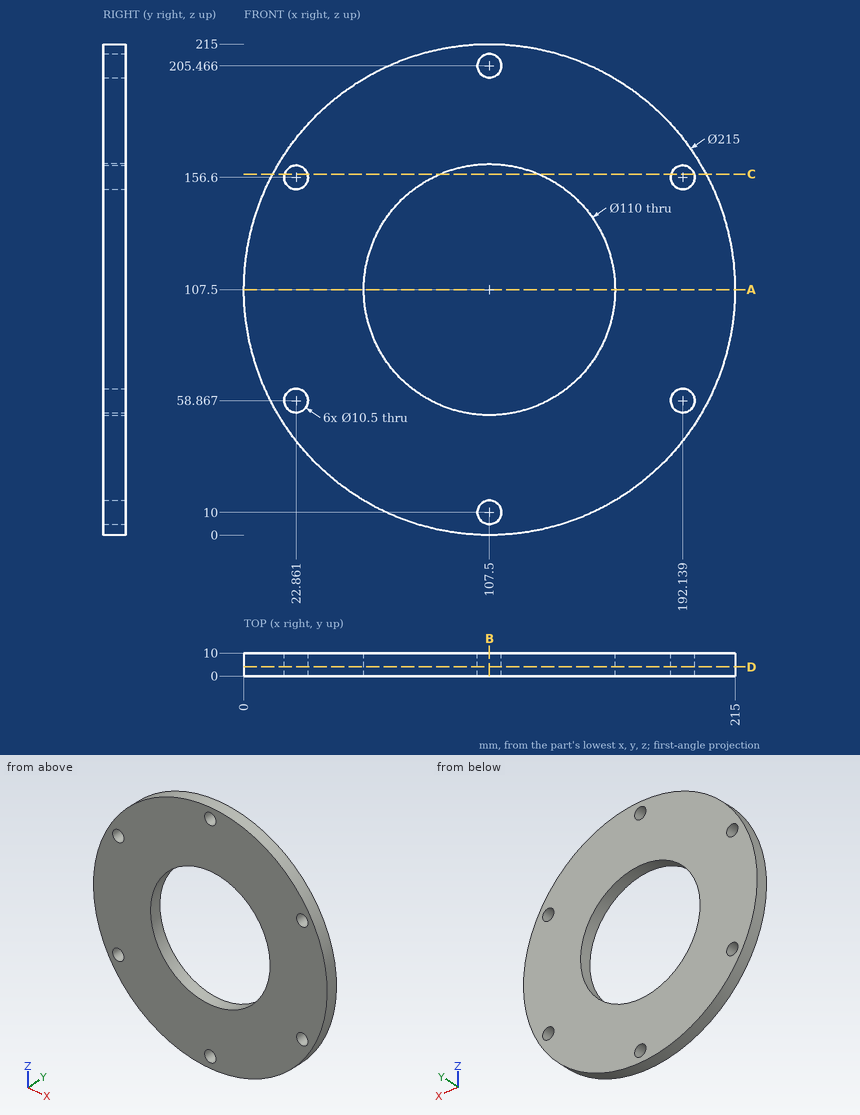
Here's the drawing with two shaded views (mm, measured from the low corner). I have some questions. Give positions to 0.01 mm unless a question says otherwise; leave off trailing zeros. Order: outer loops, then holes, each group sorted by start corner. A loop starts at its lowest first (then second) coordinate and runs counter-clockwise, first axis right, second up. Notation, with made-up numbers: (-2.75, 20) - (25.25, 20) arc R16 cw to (25.25, 43) - close; hole circle Ø5 at (29.5, 56). An arc over 180 degrees is marked (long way). Use a Markdown table: item, result. Add a question column.
Q1. If we section it at D-D on y = 4: Count the separate pieces of the cut face and the enclosed holes in it, plus the area to 3 significant figures.
Q2. I'm going to push flat-ended pins straight in: pin 1 (6 mm diameter, centred on x = 101.5, y = 7.5, fed in from -Z); pin 2 (1 mm diameter, centred on x = 114, y = 1.5, fed in from +Z); pin 3 (1 mm diameter, centred on x = 58, y = 8.5, fed in from -Z). Where does each tip first touch, or does it pass through?
Q3. If we section it at A-A on z = 107.5: Write out the boundary of the cut face in (x, y), plus the area to 3 significant figures.
Q4. Please list where these lines run through material, in increasing order: line 1 along Z through (x, y) = (108, 4.75); line 2 along X through (y, z) = (9.25, 152) (1 decimal); line 3 along Z through (x, y) = (19, 5) (1 decimal).
Q5. If we section it at B-B on x = 107.5: Write out the boundary of the cut face in (y, z), plus the area to 3 significant figures.
Q6. If we section it at C-C on z = 158: Write out the boundary of the cut face in (x, y), plus the area to 3 significant figures.
Answers follow:
| question | item | result |
|---|---|---|
| 1 | separate pieces | 1 |
| 1 | enclosed holes | 7 |
| 1 | area | 26,300 mm^2 |
| 2 | pin 1 | stops at z = 0.04 |
| 2 | pin 2 | stops at z = 214.83 |
| 2 | pin 3 | stops at z = 11.82 |
| 3 | outline | (0, 0) - (52.5, 0) - (52.5, 10) - (0, 10) - close; (162.5, 0) - (215, 0) - (215, 10) - (162.5, 10) - close |
| 3 | area | 1,050 mm^2 |
| 4 | line 1 | z = 0 to 4.77, 15.23 to 52.5, 162.5 to 200.24, 210.69 to 215 |
| 4 | line 2 | x = 9.6 to 20.3, 25.4 to 75.2, 139.8 to 189.6, 194.7 to 205.4 |
| 4 | line 3 | z = 46.5 to 55.3, 62.4 to 153, 160.2 to 168.5 |
| 5 | outline | (0, 0) - (10, 0) - (10, 4.75) - (0, 4.75) - close; (0, 15.25) - (10, 15.25) - (10, 52.5) - (0, 52.5) - close; (0, 162.5) - (10, 162.5) - (10, 200.22) - (0, 200.22) - close; (0, 210.72) - (10, 210.72) - (10, 215) - (0, 215) - close |
| 5 | area | 840 mm^2 |
| 6 | outline | (12.6, 0) - (17.8, 0) - (17.8, 10) - (12.6, 10) - close; (27.92, 0) - (85.71, 0) - (85.71, 10) - (27.92, 10) - close; (129.29, 0) - (187.08, 0) - (187.08, 10) - (129.29, 10) - close; (197.2, 0) - (202.4, 0) - (202.4, 10) - (197.2, 10) - close |
| 6 | area | 1,260 mm^2 |
